Part model, mm, in its own coordinate system. Face numbers are marked on the shaded views. A direction names the side the tool comes from. Round coordinates to 2 decimals unless told otherwise and drop trailing zeros. Order: outer loops, then holes, each group sorted by start corner. A loop starts at its lowest first (then second) coordinate and runs counter-clockwise, first axis right, second up. Notation, with made-up numbers: (-19.5, 9) - (4.5, 9) arc R18 ccw to (4.5, 22) - close; hole circle Ø11 at (58, -37.5). An arc over 180 degrees is marked (long way). Answer as a JSON object with one key per item and string values.
Autodesk Inventor part; units mm, degrees
ref_plane "YZ Plane" through (0, 0, 0) normal (1, 0, 0) x (0, 1, 0)
ref_plane "XZ Plane" through (0, 0, 0) normal (0, 1, 0) x (-1, 0, 0)
ref_plane "XY Plane" through (0, 0, 0) normal (0, 0, 1) x (1, 0, 0)
sketch "スケッチ1" plane through (0, 0, 0) normal (0, 0, 1) x (1, 0, 0)
  line L0 (-17.955, -4.955) -> (17.955, -4.955)
  line L1 (17.955, -4.955) -> (17.955, 4.955)
  line L2 (17.955, 4.955) -> (-17.955, 4.955)
  line L3 (-17.955, 4.955) -> (-17.955, -4.955)
  line L4 (-17.955, -4.955) -> (17.955, 4.955) construction
  line L5 (17.955, -4.955) -> (-17.955, 4.955) construction
  circle A0 centre (-13, 0) radius 1.55
  circle A1 centre (0, 0) radius 1.55
  line L6 (0, 0) -> (0, 4.955) construction
  line L7 (-12.5995, 4.955) -> (4.4005, 4.955) construction
  line L8 (-8.5, -4) -> (8.5, -4) construction
  line L9 (-11.2391, -3.05) -> (-14.7609, -3.05)
  line L10 (-14.7609, -3.05) -> (-16.5218, 0)
  line L11 (-16.5218, 0) -> (-14.7609, 3.05)
  line L12 (-14.7609, 3.05) -> (-11.2391, 3.05)
  line L13 (-11.2391, 3.05) -> (-9.4782, 0)
  line L14 (-9.4782, 0) -> (-11.2391, -3.05)
  circle A2 centre (-15.4718, 0) radius 1.05
  circle A3 centre (-14.2359, -2.1407) radius 1.05
  circle A4 centre (-11.7641, -2.1407) radius 1.05
  circle A5 centre (-10.5282, 0) radius 1.05
  circle A6 centre (-11.7641, 2.1407) radius 1.05
  circle A7 centre (-14.2359, 2.1407) radius 1.05
  circle A8 centre (13, 0) radius 1.55
  line L15 (11.2391, -3.05) -> (14.7609, -3.05)
  line L16 (14.7609, -3.05) -> (16.5218, 0)
  line L17 (16.5218, 0) -> (14.7609, 3.05)
  line L18 (14.7609, 3.05) -> (11.2391, 3.05)
  line L19 (11.2391, 3.05) -> (9.4782, 0)
  line L20 (9.4782, 0) -> (11.2391, -3.05)
  circle A9 centre (15.4718, 0) radius 1.05
  circle A10 centre (14.2359, -2.1407) radius 1.05
  circle A11 centre (11.7641, -2.1407) radius 1.05
  circle A12 centre (10.5282, 0) radius 1.05
  circle A13 centre (11.7641, 2.1407) radius 1.05
  circle A14 centre (14.2359, 2.1407) radius 1.05
  circle A15 centre (-13, 0) radius 4.955 construction
  line L21 (1.7609, -3.05) -> (-1.7609, -3.05)
  line L22 (-1.7609, -3.05) -> (-3.5218, 0)
  line L23 (-3.5218, 0) -> (-1.7609, 3.05)
  line L24 (-1.7609, 3.05) -> (1.7609, 3.05)
  line L25 (1.7609, 3.05) -> (3.5218, 0)
  line L26 (3.5218, 0) -> (1.7609, -3.05)
  circle A16 centre (-2.4718, 0) radius 1.05
  circle A17 centre (-1.2359, -2.1407) radius 1.05
  circle A18 centre (1.2359, -2.1407) radius 1.05
  circle A19 centre (2.4718, 0) radius 1.05
  circle A20 centre (1.2359, 2.1407) radius 1.05
  circle A21 centre (-1.2359, 2.1407) radius 1.05
  point P0 (-11.2391, -3.05)
  point P1 (-9.4782, 0)
  point P2 (-11.2391, 3.05)
  point P3 (-14.7609, 3.05)
  point P4 (11.2391, -3.05)
  point P5 (9.4782, 0)
  point P6 (11.2391, 3.05)
  point P7 (14.7609, 3.05)
  point P8 (-1.7609, -3.05)
  point P9 (1.7609, -3.05)
  point P10 (3.5218, 0)
  point P11 (1.7609, 3.05)
  point P12 (-1.7609, 3.05)
  dimension "d19" = 2.1
  dimension "d1" = 3.1
  dimension "d4" = 13
  dimension "d5" = 9.91
  dimension "d20" = 6.1
  dimension "d23" = 360
  dimension "d33" = 360
extrude "押し出し1" add sketch "スケッチ1" along normal blind 8
properties part number "胴体_サブフレーム_1_2" material "アセタール樹脂、黒"
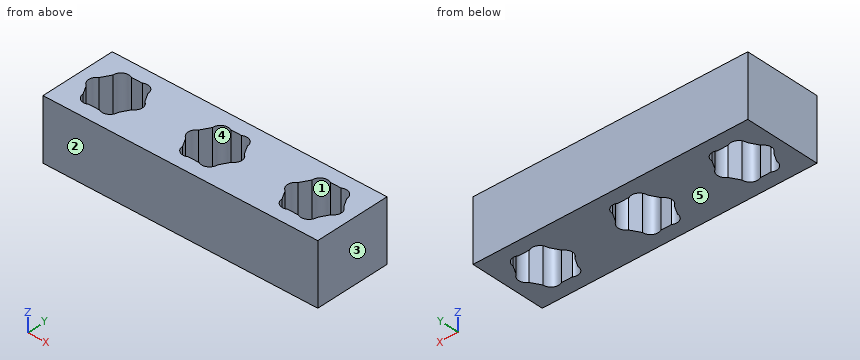
Item 1: Tool access for the marked faces 1 and 2: list every direction of +Z, -Z, +X, -X, +Y, -Y with a clear straight run to the whole face (end or side of a thin tool).
Taken from the geometry:
{"face 1": "+Z, -Z", "face 2": "+Z, -Z, +X, -X, -Y"}
Item 2: Cut at A-A (y = 1.5). Write the cut outline in (x, z) (3 decimals).
Taken from the geometry:
{"outline": "(-17.955, 0) - (-15.656, 0) - (-15.656, 8) - (-17.955, 8) - close; (-10.344, 0) - (-2.656, 0) - (-2.656, 8) - (-10.344, 8) - close; (2.656, 0) - (10.344, 0) - (10.344, 8) - (2.656, 8) - close; (15.656, 0) - (17.955, 0) - (17.955, 8) - (15.656, 8) - close"}
Item 3: Cut at B-B (z = 1). State how many separate pieces and enclosed holes the cut face has, plus the area to 3 significant figures.
Taken from the geometry:
{"separate pieces": "1", "enclosed holes": "3", "area": "256 mm2"}
Item 4: Probe L1, parallel to X at y = 0, z = 1.75 (3 decimals); L2, parallel to X at y = 2.25, z = 5.25 (3 decimals); L3, parallel to Y at x = -13.5, z = 7.75 (3 decimals). List the from-to ranges inside material, lowest first. Write a range as from..to.
Taken from the geometry:
{"L1": "-17.955..-16.522, -9.478..-3.522, 3.522..9.478, 16.522..17.955", "L2": "-17.955..-15.28, -10.72..-2.28, 2.28..10.72, 15.28..17.955", "L3": "-4.955..-3.05, 3.05..4.955"}
Item 5: Two-plate mould, pull along X, no slides. Class the marked faces 3, 4 and 5: pulls with the +X half, pulls with the -X half, needs draft (parallel to the pull), parting line crosses it, or undercut.
Taken from the geometry:
{"face 3": "pulls with the +X half", "face 4": "undercut", "face 5": "needs draft"}
